Here's how the part is built. I have some questions about the finished solid (model axes, mm). A direction names the side the tool comes from. Round coordinates to 2 decimals unless told otherwise and drop trailing zeros. Write each loop counter-clockwise with the first axis right and the second up, starting at its lowest first coordinate (ties: lowest second). Pieces come first, ordered by that corner, then holes. Notation, with made-up numbers: (22, -14.5) -> (31, -14.5) arc R6 cw to (31, -10.5) -> close; hole circle Ø5 at (59.5, 31). An arc over 180 degrees is marked (long way). Put each result on its own line as item: value. Start each with the question number.
1) I want a section at A-A, the plane z = 20. List the corners of the cut face in (x, y) for me.
2) Which directions (+Z, -Z, +X, -X, +Y, -Y) give clear straight access to the entire face, cutting with the end or side of a thin tool? Please do faces 4 (the flat face through (-1, -11, 11)), 5 (the cylindrical face through (34.8, -6.9, 11.4)).
3) Will these pins go through, and if not, where does the flat tip stop? P1, Ø10, axis at x = -14, y = -3, coming from the +Z side; P2, Ø1.8, axis at x = -36, y = 6, coming from the +Z side.
4) We'd pull the mould along X, two halves only. Please class faces 1 (the flat face through (-0.2, 10.5, 22)), 2 (the flat face through (-1, 0, 1)), 3 (the flat face through (41, 0, 11)): released by +X, released by -X, zero draft, split by the parting line, or undercut.
5) I want a section at D-D, the plane x = -36. List the corners of the cut face in (y, z) for me.
6) If I drill on line 1 along Y through (x, z) = (36, 19.6); line 2 along Y through (x, z) = (-36, 21); line 3 along X through (y, z) = (1.25, 16.5), over which ranges is the centre line in solid material (lowest first)? Write a range as [from, to].
7) I want a section at C-C, the plane y = 8.5. List the corners of the cut face in (x, z) for me, then the cut area to 3 significant figures.
8) I want a section at B-B, the plane z = 10.75. List the corners of the cut face in (x, y) for me.
from build123d import *

# Parameters (mm, degrees)
F0_W     = 80
F0_H     = 20
F0_R     = 1.5
F1_DEPTH = 1
F0_W_2   = 82
F0_H_2   = 22
F2_DEPTH = 22
F3_R     = 1
F4_DEPTH = 5
F6_DEPTH = 100


with BuildPart() as f1:
    # F0 (on Top) → F1 (new body)
    with BuildSketch(Plane.XY):
        Rectangle(F0_W, F0_H)
        with Locations((36, -6)):
            Circle(F0_R, mode=Mode.SUBTRACT)
        with Locations((-36, 6)):
            Circle(F0_R, mode=Mode.SUBTRACT)
    extrude(amount=F1_DEPTH)

    # F0 (on Top) → F2 (join)
    with BuildSketch(Plane.XY):
        Rectangle(F0_W_2, F0_H_2)
        Rectangle(F0_W, F0_H, mode=Mode.SUBTRACT)
        with Locations((-36, 6)):
            Circle(F0_R)
        with Locations((36, -6)):
            Circle(F0_R)
    extrude(amount=F2_DEPTH)

    # F3 (on face) → F4 (cut)
    with BuildSketch(Plane.XY.offset(22)):
        with Locations((36, -6)):
            Circle(F3_R)
        with Locations((-36, 6)):
            Circle(F3_R)
    extrude(amount=-F4_DEPTH, mode=Mode.SUBTRACT)

    # F5 (on face) → F6 (cut)
    with BuildSketch(Plane.YZ.offset(41)):
        with BuildLine():
            Line((-1.998466, 22), (-1.998466, 19.07831))
            ThreePointArc((-1.998466, 19.07831), (-0.023735, 17.000141), (1.999762, 19.030858))
            Line((1.999762, 19.030858), (1.999762, 22))
            Line((1.999762, 22), (-1.998466, 22))
        make_face()
    extrude(amount=-F6_DEPTH, mode=Mode.SUBTRACT)


solid = f1.part
Findings:
1. outline: (-41, -11) -> (41, -11) -> (41, -2) -> (40, -2) -> (40, -10) -> (-40, -10) -> (-40, -2) -> (-41, -2) -> close; (-41, 2) -> (-40, 2) -> (-40, 10) -> (40, 10) -> (40, 2) -> (41, 2) -> (41, 11) -> (-41, 11) -> close; circle Ø3 at (-36, 6); circle Ø3 at (36, -6); hole circle Ø2 at (-36, 6); hole circle Ø2 at (36, -6)
2. face 4: +Z, -Z, +X, -X, -Y
2. face 5: +Z
3. P1: stops at z = 1
3. P2: stops at z = 17
4. face 1: zero draft
4. face 2: undercut
4. face 3: released by +X
5. outline: (-11, 0) -> (11, 0) -> (11, 22) -> (10, 22) -> (10, 1) -> (7.5, 1) -> (7.5, 22) -> (7, 22) -> (7, 17) -> (5, 17) -> (5, 22) -> (4.5, 22) -> (4.5, 1) -> (-10, 1) -> (-10, 22) -> (-11, 22) -> close
6. line 1: y = [-11, -10], [-7.5, -7], [-5, -4.5], [10, 11]
6. line 2: y = [-11, -10], [4.5, 5], [7, 7.5], [10, 11]
6. line 3: x = [-41, -40], [40, 41]
7. outline: (-41, 0) -> (41, 0) -> (41, 22) -> (40, 22) -> (40, 1) -> (-40, 1) -> (-40, 22) -> (-41, 22) -> close
7. area: 124 mm2
8. outline: (-41, -11) -> (41, -11) -> (41, 11) -> (-41, 11) -> close; circle Ø3 at (-36, 6); circle Ø3 at (36, -6); hole (-40, -10) -> (40, -10) -> (40, 10) -> (-40, 10) -> close
